Here's how the part is built. I have some questions about the finished solid (model axes, mm). A direction names the side the tool comes from. Round coordinates to 2 decimals unless told otherwise and drop trailing zeros. Order: outer loops, then holes, each group sorted by start corner. A loop starts at its lowest first (then second) coordinate and runs counter-clockwise, first axis right, second up. Notation, with made-up numbers: (17, 62) -> (48, 62) arc R18 ccw to (48, 89) -> close; hole circle Ø1 at (72.5, 30.25). An arc over 180 degrees is marked (long way). Answer in a Markdown table with one row per item.
```python
from build123d import *

# Parameters (mm, degrees)
F1_DEPTH = 9.398


with BuildPart() as f1:
    # F0 (on Right) → F1 (new body, symmetric)
    with BuildSketch(Plane.YZ):
        with BuildLine():
            Line((-53.051602, 0), (0, 0))
            Line((0, 0), (52.764028, 0))
            Line((52.764028, 0), (54.10748, 0))
            ThreePointArc((54.10748, 0), (-2e-06, 9.859408), (-54.107483, 0))
            Line((-54.107483, 0), (-53.051602, 0))
        make_face()
        Polygon((-57.177503, -4.60484), (-53.051602, 0), (-54.107483, 0), (-55.642284, 0), (-55.642284, -1.534401), (-57.177503, -1.534401), (-57.177503, -3.069621), (-58.712725, -3.069621), (-58.712725, -4.60484), align=None)
        Polygon((54.10748, 0), (52.764028, 0), (54.10748, -1.534401), (57.149637, -4.60484), (58.668837, -4.60484), (58.668837, -3.069621), (57.149637, -3.069621), (57.149637, -1.534401), (55.630438, -1.534401), (55.630438, 0), align=None)
    extrude(amount=F1_DEPTH, both=True)


solid = f1.part
```
1. Suppose I cut it at A-A on x = -5.25. Write out the boundary of the cut face in (y, z), then the cut area to 3 significant figures.
Numbers:
| item | result |
|---|---|
| outline | (-58.71, -4.6) -> (-57.18, -4.6) -> (-53.05, 0) -> (52.76, 0) -> (54.11, -1.53) -> (57.15, -4.6) -> (58.67, -4.6) -> (58.67, -3.07) -> (57.15, -3.07) -> (57.15, -1.53) -> (55.63, -1.53) -> (55.63, 0) -> (54.11, 0) arc R153.4 ccw to (-54.11, 0) -> (-55.64, 0) -> (-55.64, -1.53) -> (-57.18, -1.53) -> (-57.18, -3.07) -> (-58.71, -3.07) -> close |
| area | 736 mm2 |
2. We'd pull the mould along Y, two halves only. Please class faces 1 (the face through (9.398, -1, 4)), 2 (the face through (0.13, -55.14, -2.33)), 3 (the face through (0.132, 0.774, 9.857)): released by +Y, released by -Y, zero draft, split by the parting line, or undercut.
Numbers:
| item | result |
|---|---|
| face 1 | zero draft |
| face 2 | undercut |
| face 3 | split by the parting line |
3. Suppose I cut it at C-C on y = -47. Write out the boundary of the cut face in (x, z), then the cut area to 3 significant figures.
Numbers:
| item | result |
|---|---|
| outline | (-9.4, 0) -> (9.4, 0) -> (9.4, 2.48) -> (-9.4, 2.48) -> close |
| area | 46.6 mm2 |
4. Please list where these lines run through material, in increasing order: line 1 along Z through (x, y) = (2.5, 0.5); line 2 along Y through (x, z) = (8.5, -0.5); line 3 along Z through (x, y) = (-6.75, 13).
Numbers:
| item | result |
|---|---|
| line 1 | z = 0 to 9.86 |
| line 2 | y = -55.64 to -53.5, 53.2 to 55.63 |
| line 3 | z = 0 to 9.31 |
5. For faces 4 (the face through (0, -1, 0)), 5 (the face through (-9.398, -1, 4)), which set-ups out of +Z, -Z, +X, -X, +Y, -Y let a thin tool reach every point of the face, with its end or its side?
Numbers:
| item | result |
|---|---|
| face 4 | -Z, +X, -X |
| face 5 | +Z, -Z, -X, +Y, -Y |
6. For pin 1 Ø0.5 at (x, y) = (-3, -56.5) entering from +Z; pin 2 Ø1.2 at (x, y) = (-0.5, -58) entering from +Z; pin 3 Ø1.5 at (x, y) = (6.5, 27) entering from +Z, each with a flat end and sliding along its axis, tell me the tip position at first contact or that it passes through.
Numbers:
| item | result |
|---|---|
| pin 1 | stops at z = -1.53 |
| pin 2 | stops at z = -3.07 |
| pin 3 | stops at z = 7.6 |
7. Suppose I cut it at B-B on z = 3. Write out the boundary of the cut face in (x, y).
Numbers:
| item | result |
|---|---|
| outline | (-9.4, -45.36) -> (9.4, -45.36) -> (9.4, 45.36) -> (-9.4, 45.36) -> close |
